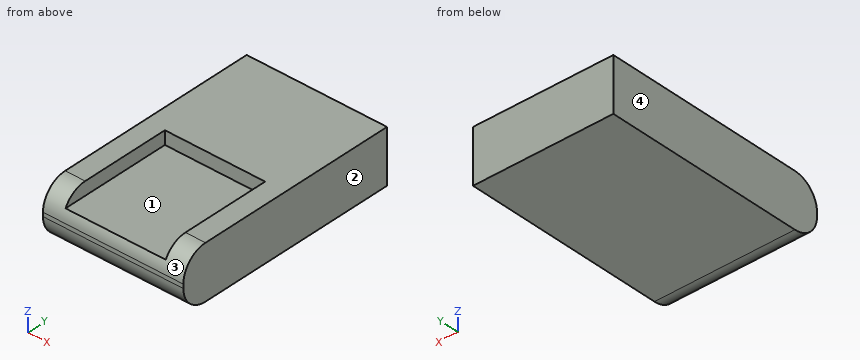
from build123d import *

# Parameters (mm, degrees)
F0_W     = 170
F0_H     = 3
F1_DEPTH = 52.5
F2_W     = 85
F2_H     = 10
F3_DEPTH = 37.5


with BuildPart() as f1:
    # F0 (on Right) → F1 (new body, symmetric)
    with BuildSketch(Plane.YZ):
        with BuildLine():
            ThreePointArc((-66.5, 20), (-79.581475, 14.581475), (-85, 1.5))
            Line((-85, 1.5), (85, 1.5))
            Line((85, 1.5), (85, 20))
            Line((85, 20), (-66.5, 20))
        make_face()
        Rectangle(F0_W, F0_H)
        with BuildLine():
            Line((85, -1.5), (-85, -1.5))
            ThreePointArc((-85, -1.5), (-79.581475, -14.581475), (-66.5, -20))
            Line((-66.5, -20), (85, -20))
            Line((85, -20), (85, -1.5))
        make_face()
    extrude(amount=F1_DEPTH, both=True)

    # F2 (on Right) → F3 (cut, symmetric)
    with BuildSketch(Plane.YZ):
        with Locations((-42.5, 15)):
            Rectangle(F2_W, F2_H)
    extrude(amount=F3_DEPTH, both=True, mode=Mode.SUBTRACT)


solid = f1.part
Source: CAD feature listing. Evaluate the final solid. Frame: model axes, mm. Face numbers are marked on the shaded views. Give positions to 0.01 mm unless a question says otherwise; leave off trailing zeros. Write each loop counter-clockwise with the first axis right and the second up, starting at its lowest first coordinate (ties: lowest second). Pieces come first, ordered by that corner, then holes. Notation, with made-up numbers: M -32.75,-11.75 L 6.25,-11.75 A11 cw 6.25,9.25 Z; hole C -5.5,14.25 d1. An arc over 180 degrees is marked long. Return JSON: item names as keys, results as strings. Group by question number.
1) Cut plane D-D, the plane z = -16.5. Output: boundary loops of the cut face in (x, y).
2) Cut plane A-A, the plane y = -31.5. Output: boundary loops of the cut face in (x, z).
3) Material intervals for line 1 along X through (y, z) = (-45.5, 18.5); line 2 along Z through (x, y) = (26.5, -33); line 3 along Y through (x, z) = (-45.5, -10), sorted ascending. Write a range as [from, to].
4) Cut plane C-C, the plane x = 44. Output: boundary loops of the cut face in (y, z), plus the area to 3 significant figures.
5) Pin query (flat end, axial travel): P1, Ø3, axis at x = 10, z = 14, coming from the -Y side; P2, Ø1.5, axis at x = -40, z = -8.5, coming from the -Y side. Return the tip coordinate at first contact, or that it passes through.
6) Pull-direction query (X, two-part tool) for the marked faces 1, 2, 3 and 4; classes: pulls with the +X half, pulls with the -X half, needs draft (parallel to the pull), parting line crosses it, or undercut.
7) Cut plane B-B, the plane z = 18. Output: boundary loops of the cut face in (x, y), plus the area to 3 significant figures.
Recorded:
{
 "1": {"outline": "M -52.5,-77.33 L 52.5,-77.33 L 52.5,85 L -52.5,85 Z"},
 "2": {"outline": "M -52.5,-20 L 52.5,-20 L 52.5,20 L 37.5,20 L 37.5,10 L -37.5,10 L -37.5,20 L -52.5,20 Z"},
 "3": {"line 1": "x = [-52.5, -37.5], [37.5, 52.5]", "line 2": "z = [-20, 10]", "line 3": "y = [-82.93, 85]"},
 "4": {"outline": "M -85,-1.5 A18.5 ccw -66.5,-20 L 85,-20 L 85,20 L -66.5,20 A18.5 ccw -85,1.5 Z", "area": "6,650 mm²"},
 "5": {"P1": "stops at y = 0", "P2": "stops at y = -83.91"},
 "6": {"face 1": "undercut", "face 2": "pulls with the +X half", "face 3": "needs draft", "face 4": "pulls with the -X half"},
 "7": {"outline": "M -52.5,-74.87 L -37.5,-74.87 L -37.5,0 L 37.5,0 L 37.5,-74.87 L 52.5,-74.87 L 52.5,85 L -52.5,85 Z", "area": "11,200 mm²"}
}
